Model file for the job. Use its own axes, mm. Face numbers are marked on the shaded views. A direction names the side the tool comes from. Give positions to 0.01 mm unless a question says otherwise; leave off trailing zeros. Write each loop counter-clockwise with the first axis right and the second up, starting at its lowest first coordinate (ties: lowest second). Pieces come first, ordered by that corner, then holes.
```python
from build123d import *

# Parameters (mm, degrees)
CUT_EXTRUDE1_DEPTH = 1


with BuildPart() as part:
    # Sketch1 → Revolve1 (revolve)
    with BuildSketch(Plane.XY):
        with BuildLine():
            Line((0, 0), (2, 0))
            Line((2, 0), (2, 10))
            Line((2, 10), (3.75, 10))
            ThreePointArc((3.75, 10), (3.043948915, 11.147830301), (2, 12))
            Line((2, 12), (0, 12))
            Line((0, 12), (0, 0))
        make_face()
    revolve(axis=Axis((0, -310.205901947, 0), (0, 1, 0)))

    # Sketch2 → Cut-Extrude1 (cut)
    with BuildSketch(Plane(origin=(0, 12, 0), x_dir=(1, 0, 0), z_dir=(0, 1, 0))):
        Polygon((2, 0), (1, 1.732050808), (-1, 1.732050808), (-2, 0), (-1, -1.732050808), (1, -1.732050808), align=None)
    extrude(amount=-CUT_EXTRUDE1_DEPTH, mode=Mode.SUBTRACT)


solid = part.part
```
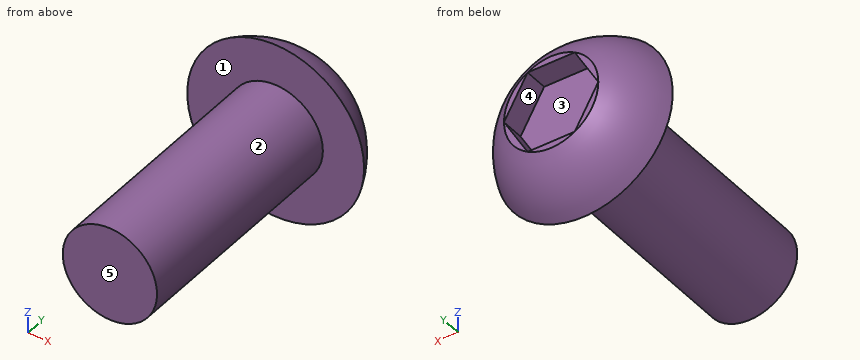
1. Which spindle directions (+Z, -Z, +X, -X, +Y, -Y) get a long thin tool onto all of the face, cutting with end or side? Do the marked faces 4 and 5. Say none if no direction does.
Calculated:
face 4: +Y
face 5: +Z, -Z, +X, -X, -Y
2. Pin check, flat tips, straight feed: P1, Ø3, axis at y = 5.5, z = 2, coming from the -X side; P2, Ø2, axis at x = -2, y = 11, coming from the +Z side; P3, Ø1.7, axis at x = 0.5, z = 0.5, coming from the +Y side. Stop position of each tip, or through.
Calculated:
P1: stops at x = -1.94
P2: stops at z = 3.39
P3: stops at y = 11
3. Slice it at C-C, the plane x = 1.5. Write the cut outline in (y, z).
Calculated:
outline: (0, -1.32) - (10, -1.32) - (10, -3.44) arc R3.76 ccw to (12, -1.32) - (12, -0.87) - (11, -0.87) - (11, 0.87) - (12, 0.87) - (12, 1.32) arc R3.76 ccw to (10, 3.44) - (10, 1.32) - (0, 1.32) - close
4. Slice it at A-A, the plane x = 0. Write the cut outline in (y, z), and give its area (3 significant figures).
Calculated:
outline: (0, -2) - (10, -2) - (10, -3.75) arc R4.04 ccw to (12, -2) - (12, -1.73) - (11, -1.73) - (11, 1.73) - (12, 1.73) - (12, 2) arc R4.04 ccw to (10, 3.75) - (10, 2) - (0, 2) - close
area: 48.8 mm2
5. Probe probe 1 along Z at (x, y) = (-1, 6.75); probe 2 along Y at (x, z) = (-2.5, 1.5). List the from-to ranges inside material, lowest first.
Calculated:
probe 1: z = -1.73 to 1.73
probe 2: y = 10 to 11.29
6. Slice it at B-B, the plane y = 6.25. Write the cut outline in (x, z).
Calculated:
outline: circle Ø4 at (0, 0)
7. Pull direction Z, two halves, no side cores. Call the marked faces 1, 2 and 3: +Z half, -Z half, draft (parallel to the pull), parting line (faces both ways), or undercut.
Calculated:
face 1: draft
face 2: parting line
face 3: undercut
